```python
from build123d import *

# Parameters (mm, degrees)
SKETCH2_W           = 30.4
SKETCH2_H           = 10.1
BOSS_EXTRUDE1_DEPTH = 8
SKETCH3_R           = 0.25
BOSS_EXTRUDE2_DEPTH = 6.3


with BuildPart() as part:
    # Sketch2 → Boss-Extrude1 (new body)
    with BuildSketch(Plane.XY):
        with Locations((15.2, 5.05)):
            Rectangle(SKETCH2_W, SKETCH2_H)
    extrude(amount=BOSS_EXTRUDE1_DEPTH)

    # Sketch3 → Boss-Extrude2 (add)
    with BuildSketch(Plane.XY.offset(8)):
        with Locations(Location((7.58, 8.805, 0), (0, 0, 180))):
            Circle(SKETCH3_R)
        with Locations(Location((10.12, 8.805, 0), (0, 0, 180))):
            Circle(SKETCH3_R)
        with Locations(Location((12.66, 8.805, 0), (0, 0, 180))):
            Circle(SKETCH3_R)
        with Locations(Location((15.2, 8.805, 0), (0, 0, 180))):
            Circle(SKETCH3_R)
        with Locations(Location((17.74, 8.805, 0), (0, 0, 180))):
            Circle(SKETCH3_R)
        with Locations(Location((20.28, 8.805, 0), (0, 0, 180))):
            Circle(SKETCH3_R)
        with Locations(Location((22.82, 8.805, 0), (0, 0, 180))):
            Circle(SKETCH3_R)
        with Locations(Location((10.12, 1.385, 0), (0, 0, 180))):
            Circle(SKETCH3_R)
        with Locations(Location((12.66, 1.385, 0), (0, 0, 180))):
            Circle(SKETCH3_R)
        with Locations(Location((15.2, 1.385, 0), (0, 0, 180))):
            Circle(SKETCH3_R)
        with Locations(Location((17.74, 1.385, 0), (0, 0, 180))):
            Circle(SKETCH3_R)
        with Locations(Location((20.28, 1.385, 0), (0, 0, 180))):
            Circle(SKETCH3_R)
        with Locations(Location((22.82, 1.385, 0), (0, 0, 180))):
            Circle(SKETCH3_R)
        with Locations(Location((7.58, 1.385, 0), (0, 0, 180))):
            Circle(SKETCH3_R)
    extrude(amount=BOSS_EXTRUDE2_DEPTH)


solid = part.part
```
Geometry check sheet. Reference: the model listing, model coordinates, mm. Give positions to 0.01 mm unless a question says otherwise; leave off trailing zeros. Write each loop counter-clockwise with the first axis right and the second up, starting at its lowest first coordinate (ties: lowest second). Pieces come first, ordered by that corner, then holes.
1) Section check A-A, the plane z = 9.5. State how many separate pieces and enclosed holes the cut face has, and give its area (3 significant figures).
2) Gauge pin test, flat ends, axial feed: pin 1 (1 mm diameter, centred on x = 10, z = 11, fed in from -Y) (3 decimals); pin 2 (6 mm diameter, centred on x = 17.5, y = 9, fed in from +Z); pin 3 (3 mm diameter, centred on x = 12.5, y = 5, fed in from +Z). Record the tip position at first contact, or that the pin passes through.
3) Material ranges on L1, parallel to Z at x = 7.5, y = 7.25; L2, parallel to Y at x = 15, z = 10 (3 decimals), recorded low to high.
4) Section check C-C, the plane x = 18.5. Record the boundary of the cut face in (y, z).
5) Section check B-B, the plane y = 9.5. Record the boundary of the cut face in (x, z), and give its area (3 significant figures).
Computed:
1. separate pieces: 14
1. enclosed holes: 0
1. area: 2.75 mm2
2. pin 1: stops at y = 1.135
2. pin 2: stops at z = 14.3
2. pin 3: stops at z = 8
3. L1: z = 0 to 8
3. L2: y = 1.235 to 1.535, 8.655 to 8.955
4. outline: (0, 0) - (10.1, 0) - (10.1, 8) - (0, 8) - close
5. outline: (0, 0) - (30.4, 0) - (30.4, 8) - (0, 8) - close
5. area: 243 mm2
